```python
from build123d import *

# Parameters (mm, degrees)
F0_W     = 80
F0_H     = 90
F1_DEPTH = 20
F2_W     = 71
F2_H     = 83.6
F3_DEPTH = 17
F4_W     = 16
F4_H     = 3.2
F5_DEPTH = 17
F6_R     = 5


with BuildPart() as f1:
    # F0 (on Top) → F1 (new body)
    with BuildSketch(Plane.XY):
        Rectangle(F0_W, F0_H)
    extrude(amount=F1_DEPTH)

    # F2 (on face) → F3 (cut)
    with BuildSketch(Plane.XY.offset(20)):
        Rectangle(F2_W, F2_H)
    extrude(amount=-F3_DEPTH, mode=Mode.SUBTRACT)

    # F4 (on face) → F5 (cut, through all)
    with BuildSketch(Plane.XY.offset(20)):
        with Locations((12.5, 43.4)):
            Rectangle(F4_W, F4_H)
    extrude(amount=-F5_DEPTH, mode=Mode.SUBTRACT)

    # F6
    f6_edges = [f1.edges().sort_by_distance(p)[0] for p in [
        (40, 45, 10),
        (-40, 45, 10),
        (40, -45, 10),
        (-40, -45, 10),
    ]]
    fillet(f6_edges, radius=F6_R)


solid = f1.part
```
Check sheet for the modelled part. Datum: model origin and axes. Units: mm. A direction names the side the tool comes from. Round coordinates to 2 decimals unless told otherwise and drop trailing zeros. Order: outer loops, then holes, each group sorted by start corner. A loop starts at its lowest first (then second) coordinate and runs counter-clockwise, first axis right, second up. Notation, with made-up numbers: (23, 0) -> (31, 0) arc R18 cw to (31, 32) -> close; hole circle Ø2 at (9.5, 87). An arc over 180 degrees is marked (long way). Use CSV: the item, a comma, the result in double quotes.
(1) Material ranges on line 1 along Y through (x, z) = (24, 11.75); line 2 along X through (y, z) = (-38, 8.5); line 3 along Z through (x, y) = (-3, 34), recorded low to high. Write a range as from..to.
Worked out:
line 1,"-45..-41.8, 41.8..45"
line 2,"-40..-35.5, 35.5..40"
line 3,"0..3"
(2) Draft check along X on faces 4 (the face through (38, -44, 10)), 5 (the face through (-40, -1, 10)), 6 (the face through (0, -45, 10)), 7 (the face through (35.5, -1, 12)). Enter one of: pulls with the +X half, pulls with the -X half, needs draft (parallel to the pull), parting line crosses it, or undercut.
Worked out:
face 4,"pulls with the +X half"
face 5,"pulls with the -X half"
face 6,"needs draft"
face 7,"undercut"
(3) Cross-section at A-A (y = 20). Record the boundary of the cut face in (x, z).
Worked out:
outline,"(-40, 0) -> (40, 0) -> (40, 20) -> (35.5, 20) -> (35.5, 3) -> (-35.5, 3) -> (-35.5, 20) -> (-40, 20) -> close"
(4) Cross-section at B-B (x = -20). Record the boundary of the cut face in (y, z).
Worked out:
outline,"(-45, 0) -> (45, 0) -> (45, 20) -> (41.8, 20) -> (41.8, 3) -> (-41.8, 3) -> (-41.8, 20) -> (-45, 20) -> close"
(5) Depth check by flat-ended pin: pin 1 (2 mm diameter, centred on x = 8.5, z = 8.5, fed in from +Y); pin 2 (4 mm diameter, centred on x = 21.5, y = 7.5, fed in from +Z); pin 3 (3.5 mm diameter, centred on y = 44, z = 12, fed in from -X). Enter the tip coordinate at first touch or a pass-through.
Worked out:
pin 1,"y = -41.8"
pin 2,"z = 3"
pin 3,"x = -39.47"
(6) Cross-section at D-D (x = 15.5). Record the boundary of the cut face in (y, z), and give its area (3 significant figures).
Worked out:
outline,"(-45, 0) -> (45, 0) -> (45, 3) -> (-41.8, 3) -> (-41.8, 20) -> (-45, 20) -> close"
area,"324 mm²"
(7) Tool access check on faces 1 (the face through (-39, -43, 10)), 2 (the face through (20.5, 43, 12)), 3 (the face through (-16, 41.8, 12)). Record the directions out of +Z, -Z, +X, -X, +Y, -Y that give a thin tool (end or side, any length) a straight path to the whole face; none if there is none.
Worked out:
face 1,"+Z, -Z, -X, -Y"
face 2,"+Z, +Y"
face 3,"+Z"
(8) Cross-section at C-C (z = 9.25). Record the boundary of the cut face in (x, y).
Worked out:
outline,"(-40, -40) arc R5 ccw to (-35, -45) -> (35, -45) arc R5 ccw to (40, -40) -> (40, 40) arc R5 ccw to (35, 45) -> (20.5, 45) -> (20.5, 41.8) -> (35.5, 41.8) -> (35.5, -41.8) -> (-35.5, -41.8) -> (-35.5, 41.8) -> (4.5, 41.8) -> (4.5, 45) -> (-35, 45) arc R5 ccw to (-40, 40) -> close"
